The listing builds one solid part. Answer for the finished solid, in the listing's coordinates (mm). A direction names the side the tool comes from. Round coordinates to 2 decimals unless told otherwise and drop trailing zeros. Loops run counter-clockwise (first coordinate to the right, second up) from the corner with the lowest first, then second, coordinate; pieces in that order, holes last. Notation, with made-up numbers: (5, 52.25) -> (64, 52.25) arc R36 cw to (64, 90.25) -> close; hole circle Ø10 at (11, -32.5). An arc over 180 degrees is marked (long way). Write each question's results on one line, items separated by ' | '. Start each with the question number.
(1) The part is cut by section C-C (x = -20.5). Determine the outline of the cut face in (y, z), plus the area to 3 significant figures.
(2) The part is cut by section D-D (y = 8.5). Determine the outline of the cut face in (x, z), plus the area to 3 significant figures.
(3) Straight lines are drawn through the part: probe 1 along Z at (x, y) = (23.5, -1.5); probe 2 along Z at (x, y) = (29.5, 9.25); probe 3 along X at (y, z) = (8.5, 4.5). For each, find the intervals that lie inside material, in ascending order.
(4) The part is cut by section A-A (y = -1.75). Determine the outline of the cut face in (x, z), plus the area to 4 significant figures.
(5) Determine the mould class of faces 1 (the face through (-1, -2, 4.4)), 2 (the face through (-1, -2, 8.9)), 3 (the face through (35.25, 8, 0)), 4 (the face through (37, 14, -4)) for opening direction Z: released by +Z, released by -Z, zero draft, split by the parting line, or undercut.
(6) For faces 5 (the face through (37, 9, -13.15)), 6 (the face through (38.25, 4, 0)), 7 (the face through (0, 8, -27.25)), 8 (the face through (-1, -4.8, 7)), 9 (the face through (-1, 0, -20)), determine the directions among +Z, -Z, +X, -X, +Y, -Y from which every point of the face is accessible in a straight line to the end or side of a thin tool.
(7) The part is cut by section B-B (z = -18.97). Determine the outline of the cut face in (x, y).
(8) Flat-ended cylindrical pins translate along their axes: pin 1 (1 mm diameter, centred on y = -1.5, z = 22, fed in from -X); pin 2 (4 mm diameter, centred on x = -27, z = -0.5, fed in from -Y); pin 3 (2.5 mm diameter, centred on x = 12.5, y = -2.5, fed in from -Z); pin 4 (3 mm diameter, centred on x = -30.5, z = -18.5, fed in from +Y). Find the tip coordinate at first contact, or state that the pin passes through.
```python
from build123d import *

# Parameters (mm, degrees)
SKETCH1_W           = 76.5
SKETCH1_H           = 60.5
BOSS_EXTRUDE1_DEPTH = 14
SKETCH2_W           = 70.5
SKETCH2_H           = 54.5
CUT_EXTRUDE1_DEPTH  = 12
CUT_EXTRUDE2_REACH  = 85.446
SKETCH4_W           = 13
SKETCH4_H           = 9
SKETCH4_W_2         = 10.2
SKETCH5_W           = 76.5
SKETCH5_H           = 4.5
BOSS_EXTRUDE3_DEPTH = 4.8
SKETCH6_R           = 1.4
BOSS_EXTRUDE4_DEPTH = 5


with BuildPart() as part:
    # Sketch1 → Boss-Extrude1 (new body)
    with BuildSketch(Plane(origin=(0, 0, 0), x_dir=(1, 0, 0), z_dir=(0, 1, 0))):
        Rectangle(SKETCH1_W, SKETCH1_H)
    extrude(amount=BOSS_EXTRUDE1_DEPTH)

    # Sketch2 → Cut-Extrude1 (cut)
    with BuildSketch(Plane(origin=(0, 14, 0), x_dir=(1, 0, 0), z_dir=(0, 1, 0))):
        Rectangle(SKETCH2_W, SKETCH2_H)
    extrude(amount=-CUT_EXTRUDE1_DEPTH, mode=Mode.SUBTRACT)

    # Sketch4 → Cut-Extrude2 (cut, up to next)
    with BuildSketch(Plane(origin=(38.25, 0, 0), x_dir=(0, 0, -1), z_dir=(1, 0, 0)), mode=Mode.PRIVATE) as cut_extrude2_sk1:
        with Locations((-11.85, 9.5)):
            Rectangle(SKETCH4_W, SKETCH4_H)
    cut_extrude2_tool1 = extrude(cut_extrude2_sk1.sketch, amount=-CUT_EXTRUDE2_REACH, mode=Mode.PRIVATE) & part.part
    # Sketch4 → Cut-Extrude2 (cut, up to next)
    with BuildSketch(Plane(origin=(38.25, 0, 0), x_dir=(0, 0, -1), z_dir=(1, 0, 0)), mode=Mode.PRIVATE) as cut_extrude2_sk2:
        with Locations((18.25, 9.5)):
            Rectangle(SKETCH4_W_2, SKETCH4_H)
    cut_extrude2_tool2 = extrude(cut_extrude2_sk2.sketch, amount=-CUT_EXTRUDE2_REACH, mode=Mode.PRIVATE) & part.part
    add(cut_extrude2_tool1.solids().sort_by_distance((38.25, 9.5, 11.85))[0], mode=Mode.SUBTRACT)
    add(cut_extrude2_tool2.solids().sort_by_distance((38.25, 9.5, -18.25))[0], mode=Mode.SUBTRACT)

    # Sketch5 → Boss-Extrude3 (add)
    with BuildSketch(Plane.XZ):
        with Locations((0, 6.65)):
            Rectangle(SKETCH5_W, SKETCH5_H)
    boss_extrude3 = extrude(amount=BOSS_EXTRUDE3_DEPTH)

    # Mirror1: Boss-Extrude3 across plane
    add(boss_extrude3.mirror(Plane.XY))

    # Sketch6 → Boss-Extrude4 (add)
    with BuildSketch(Plane(origin=(0, 2, 0), x_dir=(1, 0, 0), z_dir=(0, 1, 0))):
        with Locations(Location((-31.29, -8.97, 0), (0, 0, 270))):
            Circle(SKETCH6_R)
        with Locations(Location((-31.29, 18.97, 0), (0, 0, 270))):
            Circle(SKETCH6_R)
    extrude(amount=BOSS_EXTRUDE4_DEPTH)


solid = part.part
```
Checked values:
1) outline: (-4.8, -8.9) -> (0, -8.9) -> (0, -30.25) -> (14, -30.25) -> (14, -27.25) -> (2, -27.25) -> (2, 27.25) -> (14, 27.25) -> (14, 30.25) -> (0, 30.25) -> (0, 8.9) -> (-4.8, 8.9) -> (-4.8, 4.4) -> (0, 4.4) -> (0, -4.4) -> (-4.8, -4.4) -> close | area: 236 mm2
2) outline: (-38.25, -30.25) -> (38.25, -30.25) -> (38.25, -23.35) -> (35.25, -23.35) -> (35.25, -27.25) -> (-35.25, -27.25) -> (-35.25, 27.25) -> (35.25, 27.25) -> (35.25, 18.35) -> (38.25, 18.35) -> (38.25, 30.25) -> (-38.25, 30.25) -> close; (35.25, -13.15) -> (38.25, -13.15) -> (38.25, 5.35) -> (35.25, 5.35) -> close | area: 716 mm2
3) probe 1: z = -8.9 to -4.4, 4.4 to 8.9 | probe 2: z = -30.25 to -27.25, 27.25 to 30.25 | probe 3: x = -38.25 to -35.25, 35.25 to 38.25
4) outline: (-38.25, -8.9) -> (38.25, -8.9) -> (38.25, -4.4) -> (-38.25, -4.4) -> close; (-38.25, 4.4) -> (38.25, 4.4) -> (38.25, 8.9) -> (-38.25, 8.9) -> close | area: 688.5 mm2
5) face 1: undercut | face 2: released by +Z | face 3: undercut | face 4: zero draft
6) face 5: +X, +Y | face 6: +Z, -Z, +X, +Y, -Y | face 7: +Y | face 8: +Z, -Z, +X, -X, -Y | face 9: -Z, +X, -X, -Y
7) outline: (-38.25, 0) -> (38.25, 0) -> (38.25, 5) -> (35.25, 5) -> (35.25, 2) -> (-29.89, 2) -> (-29.89, 7) -> (-32.69, 7) -> (-32.69, 2) -> (-35.25, 2) -> (-35.25, 14) -> (-38.25, 14) -> close
8) pin 1: passes through | pin 2: stops at y = 0 | pin 3: stops at z = -8.9 | pin 4: stops at y = 7
